Input: part model. Units: mm. Frame: model coordinates. A direction names the side the tool comes from. Round coordinates to 2 decimals unless told otherwise and drop trailing zeros. Order: outer loops, then holes, each group sorted by start corner. A loop starts at its lowest first (then second) coordinate and runs counter-clockwise, first axis right, second up.
Item 1: Cut plane B-B on z = 19.05. Output: boundary loops of the cut face in (x, y), then the cut area to 3 significant figures.
Item 2: Cut plane A-A on z = 38.1. Output: boundary loops of the cut face in (x, y), then the cut area to 3 significant figures.
Item 3: First-contact query: pin 1 (1 mm diameter, centred on x = 3, z = 19.5, fed in from +Y); pin 2 (5 mm diameter, centred on x = 10.32, z = 38.1, fed in from +Y); pin 3 (14 mm diameter, centred on y = 13, z = 20.5, fed in from +X). Flat tips, straight axial feed; report the tip coordinate or a pass-through.
Item 4: Reachability of faces 1 (the flat face through (6, 0, 38)), 2 (the cylindrical face through (7.22, -2.35, 37.41)) from +Z, -Z, +X, -X, +Y, -Y: full face, straight path, thin tool, end or side. Return the list, or none.
Item 5: Mould query, pull axis X, two halves, no side actions, for faces 3 (the cylindrical face through (11.27, -2.35, 66.53)), 4 (the flat face through (-1, 15, 76.2)), 5 (the cylindrical face through (8.39, -2.35, 10.18)), 6 (the flat face through (-4.762, 21, 38)). Classes: released by +X, released by -X, zero draft, split by the parting line, or undercut.
Item 6: Cut plane C-C on y = 31. Output: boundary loops of the cut face in (x, z).
Item 7: Cut plane D-D on z = 48.5. Output: boundary loops of the cut face in (x, y).
Item 8: Line query: L1, parallel to Y at x = -2, z = 19.05; L2, parallel to X at y = 7, z = 40. Output: solid intervals per line, ascending.
```python
from build123d import *

# Parameters (mm, degrees)
BOSS_EXTRUDE1_DEPTH = 76.2
CUT_EXTRUDE1_REACH  = 93.388
SKETCH2_R           = 3.175
CUT_EXTRUDE2_REACH  = 93.388
SKETCH3_R           = 3.175


with BuildPart() as part:
    # Sketch1 → Boss-Extrude1 (new body)
    with BuildSketch(Plane.XY):
        Polygon((0, 0), (0, 46.0375), (-4.7625, 46.0375), (-4.7625, -4.7625), (20.6375, -4.7625), (20.6375, 0), align=None)
    extrude(amount=BOSS_EXTRUDE1_DEPTH)

    # Sketch2 → Cut-Extrude1 (cut, up to next)
    with BuildSketch(Plane(origin=(0, 0, 0), x_dir=(0, 0, -1), z_dir=(1, 0, 0)), mode=Mode.PRIVATE) as cut_extrude1_sk1:
        with Locations((-57.15, 33.3375)):
            Circle(SKETCH2_R)
    cut_extrude1_tool1 = extrude(cut_extrude1_sk1.sketch, amount=-CUT_EXTRUDE1_REACH, mode=Mode.PRIVATE) & part.part
    # Sketch2 → Cut-Extrude1 (cut, up to next)
    with BuildSketch(Plane(origin=(0, 0, 0), x_dir=(0, 0, -1), z_dir=(1, 0, 0)), mode=Mode.PRIVATE) as cut_extrude1_sk2:
        with Locations((-19.05, 33.3375)):
            Circle(SKETCH2_R)
    cut_extrude1_tool2 = extrude(cut_extrude1_sk2.sketch, amount=-CUT_EXTRUDE1_REACH, mode=Mode.PRIVATE) & part.part
    # Sketch2 → Cut-Extrude1 (cut, up to next)
    with BuildSketch(Plane(origin=(0, 0, 0), x_dir=(0, 0, -1), z_dir=(1, 0, 0)), mode=Mode.PRIVATE) as cut_extrude1_sk3:
        with Locations((-19.05, 14.2875)):
            Circle(SKETCH2_R)
    cut_extrude1_tool3 = extrude(cut_extrude1_sk3.sketch, amount=-CUT_EXTRUDE1_REACH, mode=Mode.PRIVATE) & part.part
    # Sketch2 → Cut-Extrude1 (cut, up to next)
    with BuildSketch(Plane(origin=(0, 0, 0), x_dir=(0, 0, -1), z_dir=(1, 0, 0)), mode=Mode.PRIVATE) as cut_extrude1_sk4:
        with Locations((-57.15, 14.2875)):
            Circle(SKETCH2_R)
    cut_extrude1_tool4 = extrude(cut_extrude1_sk4.sketch, amount=-CUT_EXTRUDE1_REACH, mode=Mode.PRIVATE) & part.part
    add(cut_extrude1_tool1.solids().sort_by_distance((0, 33.3375, 57.15))[0], mode=Mode.SUBTRACT)
    add(cut_extrude1_tool2.solids().sort_by_distance((0, 33.3375, 19.05))[0], mode=Mode.SUBTRACT)
    add(cut_extrude1_tool3.solids().sort_by_distance((0, 14.2875, 19.05))[0], mode=Mode.SUBTRACT)
    add(cut_extrude1_tool4.solids().sort_by_distance((0, 14.2875, 57.15))[0], mode=Mode.SUBTRACT)

    # Sketch3 → Cut-Extrude2 (cut, up to next)
    with BuildSketch(Plane(origin=(0, 0, 0), x_dir=(1, 0, 0), z_dir=(0, 1, 0)), mode=Mode.PRIVATE) as cut_extrude2_sk1:
        with Locations(Location((10.31875, -12.7, 0), (0, 0, 270))):
            Circle(SKETCH3_R)
    cut_extrude2_tool1 = extrude(cut_extrude2_sk1.sketch, amount=-CUT_EXTRUDE2_REACH, mode=Mode.PRIVATE) & part.part
    # Sketch3 → Cut-Extrude2 (cut, up to next)
    with BuildSketch(Plane(origin=(0, 0, 0), x_dir=(1, 0, 0), z_dir=(0, 1, 0)), mode=Mode.PRIVATE) as cut_extrude2_sk2:
        with Locations(Location((10.31875, -63.5, 0), (0, 0, 270))):
            Circle(SKETCH3_R)
    cut_extrude2_tool2 = extrude(cut_extrude2_sk2.sketch, amount=-CUT_EXTRUDE2_REACH, mode=Mode.PRIVATE) & part.part
    # Sketch3 → Cut-Extrude2 (cut, up to next)
    with BuildSketch(Plane(origin=(0, 0, 0), x_dir=(1, 0, 0), z_dir=(0, 1, 0)), mode=Mode.PRIVATE) as cut_extrude2_sk3:
        with Locations(Location((10.31875, -38.1, 0), (0, 0, 270))):
            Circle(SKETCH3_R)
    cut_extrude2_tool3 = extrude(cut_extrude2_sk3.sketch, amount=-CUT_EXTRUDE2_REACH, mode=Mode.PRIVATE) & part.part
    add(cut_extrude2_tool1.solids().sort_by_distance((10.31875, 0, 12.7))[0], mode=Mode.SUBTRACT)
    add(cut_extrude2_tool2.solids().sort_by_distance((10.31875, 0, 63.5))[0], mode=Mode.SUBTRACT)
    add(cut_extrude2_tool3.solids().sort_by_distance((10.31875, 0, 38.1))[0], mode=Mode.SUBTRACT)


solid = part.part
```
From the geometry:
1. outline: (-4.76, -4.76) - (20.64, -4.76) - (20.64, 0) - (0, 0) - (0, 11.11) - (-4.76, 11.11) - close; (-4.76, 17.46) - (0, 17.46) - (0, 30.16) - (-4.76, 30.16) - close; (-4.76, 36.51) - (0, 36.51) - (0, 46.04) - (-4.76, 46.04) - close
1. area: 280 mm2
2. outline: (-4.76, -4.76) - (7.14, -4.76) - (7.14, 0) - (0, 0) - (0, 46.04) - (-4.76, 46.04) - close; (13.49, -4.76) - (20.64, -4.76) - (20.64, 0) - (13.49, 0) - close
2. area: 310 mm2
3. pin 1: stops at y = 0
3. pin 2: passes through
3. pin 3: stops at x = 0
4. face 1: +Z, -Z, +X, +Y
4. face 2: +Y, -Y
5. face 3: undercut
5. face 4: zero draft
5. face 5: undercut
5. face 6: released by -X
6. outline: (-4.76, 0) - (0, 0) - (0, 16.9) - (-4.76, 16.9) - close; (-4.76, 21.2) - (0, 21.2) - (0, 55) - (-4.76, 55) - close; (-4.76, 59.3) - (0, 59.3) - (0, 76.2) - (-4.76, 76.2) - close
7. outline: (-4.76, -4.76) - (20.64, -4.76) - (20.64, 0) - (0, 0) - (0, 46.04) - (-4.76, 46.04) - close
8. L1: y = -4.76 to 11.11, 17.46 to 30.16, 36.51 to 46.04
8. L2: x = -4.76 to 0
